Answer from the drawing. Dimensions are ordinates in mm from the lowest x, y and z of the part. Round coordinates to 2 decimals unless told otherwise and drop trailing zeros. Loops run counter-clockwise (first coordinate to the right, second up) from the corner with the lowest first, then second, coordinate; pieces in that order, holes last. Notation, with made-up numbers: (84, 33) - (138, 33) arc R12 cw to (138, 55) - close; hole circle Ø1 at (-15, 73). An arc over 180 degrees is marked (long way). Answer as CSV lines item,"result". Start each with the question number.
Q1. Straight lines are drawn through the part: L1, parallel to Z at x = 22, y = 5; L2, parallel to X at y = 27, z = 10.5. For each, find the intervals that lie inside material, in ascending order. Write a range as [from, to].
Q2. Each of these flat-tipped pins is pushed along its axis until it touches: pin 1 Ø1 at (y, z) = (10.5, 11.5) entering from +X; pin 2 Ø7 at (x, z) = (13.5, 12.5) entering from +Y. Where does it stop, or does it pass through?
Q3. Section C-C on z = 8.75 is taken. Write down the section's boundary in (x, y), then the cut area to 3 significant figures.
Q4. Section B-B on y = 27 is taken. Write down the section's boundary in (x, z).
Q5. The mould has two halves that part along Z. Classify the marked faces 1, 2 and 3: +Z half, -Z half, draft (parallel to the pull), parting line (faces both ways), or undercut.
Q6. Section A-A on x = 11 is taken. Write down the section's boundary in (y, z).
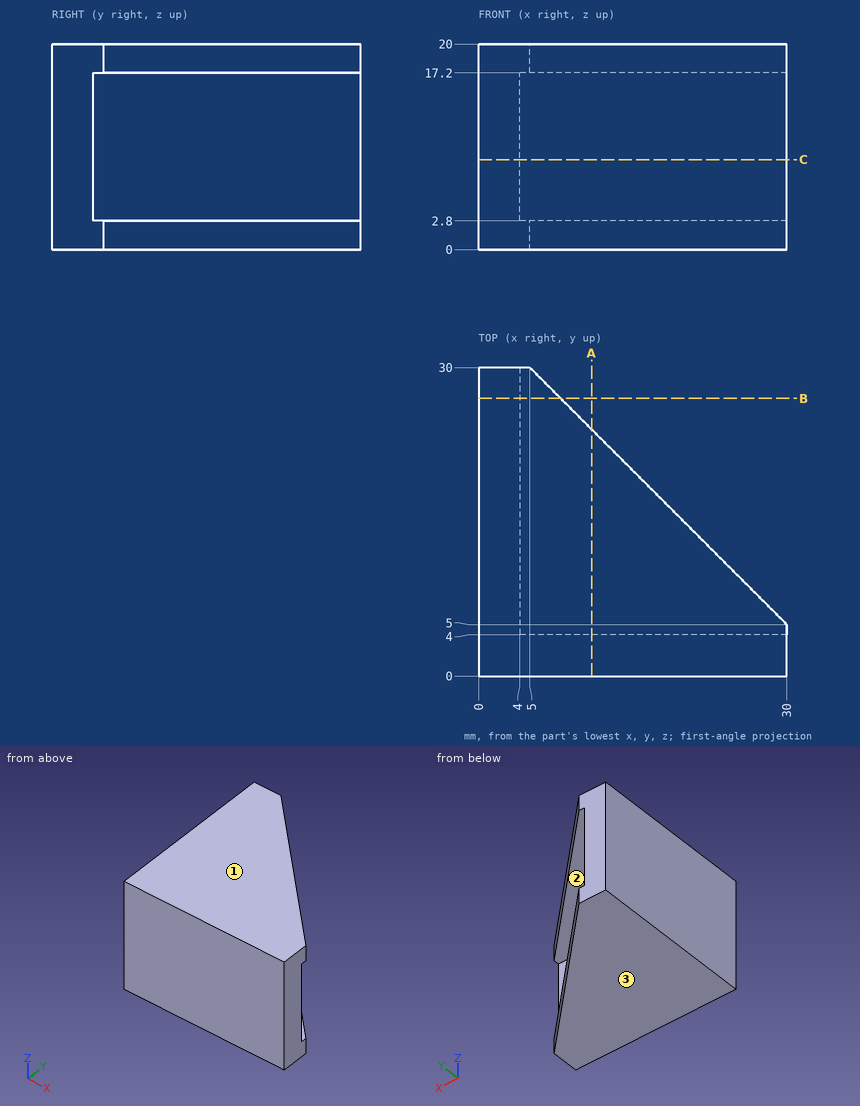
Findings:
1,L1,"z = [0, 2.8], [17.2, 20]"
1,L2,"x = [0, 4]"
2,pin 1,"stops at x = 4"
2,pin 2,"stops at y = 4"
3,outline,"(0, 0) - (30, 0) - (30, 4) - (4, 4) - (4, 30) - (0, 30) - close"
3,area,"224 mm^2"
4,outline,"(0, 0) - (8, 0) - (8, 2.8) - (4, 2.8) - (4, 17.2) - (8, 17.2) - (8, 20) - (0, 20) - close"
5,face 1,"+Z half"
5,face 2,"undercut"
5,face 3,"-Z half"
6,outline,"(0, 0) - (24, 0) - (24, 2.8) - (4, 2.8) - (4, 17.2) - (24, 17.2) - (24, 20) - (0, 20) - close"
